The drawing under review shows one solid part. Ordinate dimensions are in mm from its lowest x, y, z. A direction names the side the tool comes from. Give positions to 0.01 mm unless a question says otherwise; leave off trailing zeros. Write each loop counter-clockwise with the first axis right and the second up, starting at its lowest first coordinate (ties: lowest second). Pieces come first, ordered by that corner, then holes. Notation, with made-up numbers: M 65,-2 L 106,-2 A17 ccw 106,16 Z; hole C 88.5,9 d1. An arc over 180 degrees is marked long. Use one line per item in the form item = value. Start each with the question number.
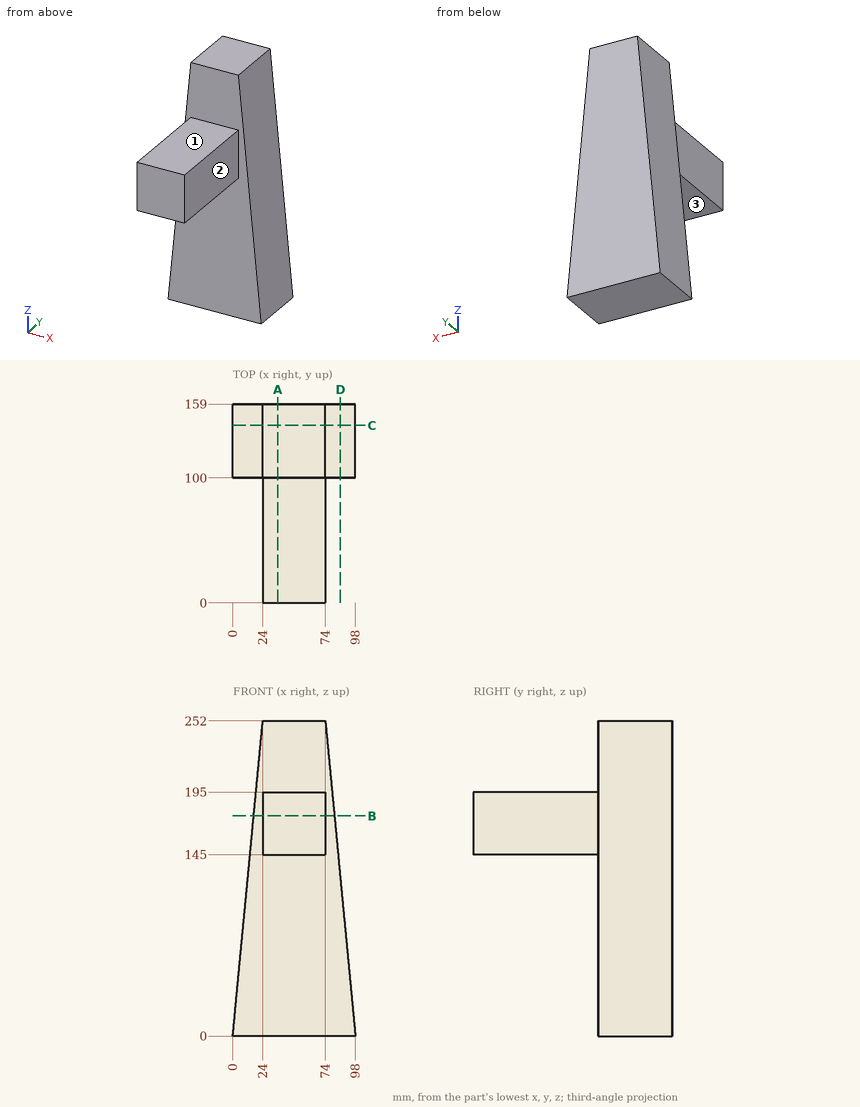
1. We need section B-B (z = 176). State the section outline as (x, y) points, and give its area (3 significant figures).
2. To check wall thickness, follow L1, parallel to Y at x = 42, z = 195.5; L2, parallel to Z at x = 24.5, y = 85; L3, parallel to X at y = 16, z = 157.5. State the ranges of each line that lie inside material, in increasing order.
3. We need section C-C (y = 142). State the section outline as (x, z) points.
4. We need section A-A (x = 36). State the section outline as (y, z) points.
5. Clearance check with flat-ended pins moving along their axes: pin 1 Ø4 at (y, z) = (130.5, 219) entering from -X; pin 2 Ø1 at (y, z) = (69, 156) entering from -X; pin 3 Ø12 at (y, z) = (60, 153.5) entering from +X. State where each tip first meets the part, or that it passes through.
6. For the marked faces 1, 2 and 3, list the 3-axis set-ups (+Z, -Z, +X, -X, +Y, -Y) from which the entire face can be reached by the end or side of a thin tool; tool diameter is ignored.
7. We need section D-D (x = 86). State the section outline as (y, z) points.
Answer block:
q1.outline = M 16.76,100 L 24,100 L 24,0 L 74,0 L 74,100 L 81.24,100 L 81.24,159 L 16.76,159 Z
q1.area = 8,800 mm^2
q2.L1 = 100 to 159
q2.L2 = 145 to 195
q2.L3 = 24 to 74
q3.outline = M 0,0 L 98,0 L 74,252 L 24,252 Z
q4.outline = M 0,145 L 100,145 L 100,0 L 159,0 L 159,252 L 100,252 L 100,195 L 0,195 Z
q5.pin_1 = 20.67
q5.pin_2 = 24
q5.pin_3 = 74
q6.face_1 = +Z, +X, -X, -Y
q6.face_2 = +Z, -Z, +X, -Y
q6.face_3 = -Z, +X, -X, -Y
q7.outline = M 100,0 L 159,0 L 159,126 L 100,126 Z
